Check sheet for the drawn part. Datum: minimum x, y, z corner. Units: mm. A direction names the side the tool comes from. Round coordinates to 2 decimals unless told otherwise and drop trailing zeros. Write each loop counter-clockwise with the first axis right and the second up, starting at its lowest first coordinate (ties: lowest second). Pieces come first, ordered by that corner, then holes. Notation, with made-up numbers: M 51.25,52.25 L 97.25,52.25 A23 cw 97.25,80.25 Z; hole C 49,58 d4. An arc over 180 degrees is marked long. One line per item, written item: value. Start each with the question number.
Item 1: Section check D-D, the plane x = 57.5. Record the cut outline in (y, z) (1 decimal).
Item 2: Section check C-C, the plane z = 24.5. Record the cut outline in (x, y), then the cut area to 3 significant figures.
Item 3: Thickness scan on probe 1 along Y at (x, z) = (97, 122); probe 2 along Z at (x, y) = (96, 33); probe 3 along X at (y, z) = (84, 38.5). Record the ranges inside material, lowest first. Write a range as from..to.
Item 4: Gauge pin test, flat ends, axial feed: pin 1 (10 mm diameter, centred on x = 66.5, y = 100.5, fed in from +Z); pin 2 (23 mm diameter, centred on x = 17.5, y = 20, fed in from -Z); pin 3 (5 mm diameter, centred on y = 39.5, z = 32.5, fed in from +X). Record the tip position at first contact, or that the pin passes through.
Item 5: Tool access check on the marked faces 1, 2, 3, 4 and 5. Record the directions out of +Z, -Z, +X, -X, +Y, -Y that give a thin tool (end or side, any length) a straight path to the whole face; none if there is none.
Item 6: Section check A-A, the plane x = 97.5. Record the cut outline in (y, z), then the cut area to 3 significant figures.
Item 7: Section check B-B, the plane y = 20. Record the cut outline in (x, z).
Item 8: Draft check along Y on the marked faces 6, 7 and 8. Enter one of: +Y half, -Y half, draft (parallel to the pull), parting line (faces both ways), or undercut.
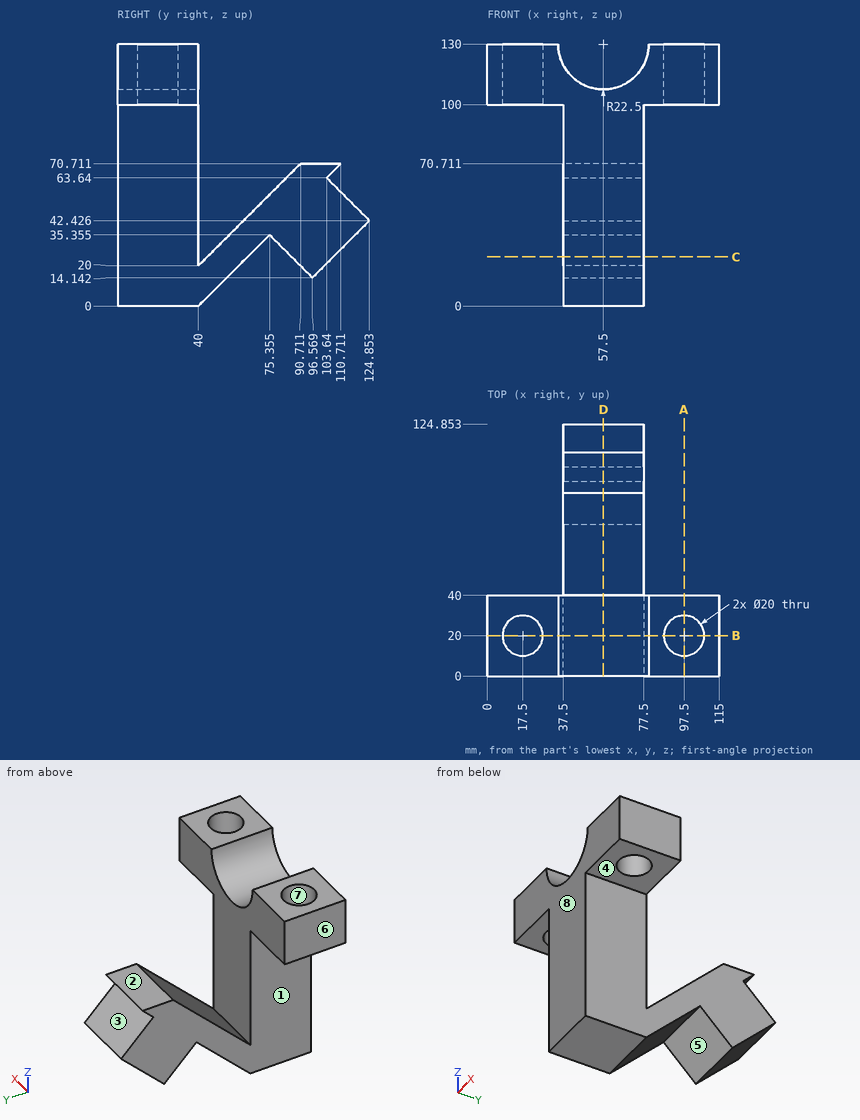
Response values:
1. outline: M 0,0 L 40,0 L 75.4,35.4 L 96.6,14.1 L 124.9,42.4 L 103.6,63.6 L 110.7,70.7 L 90.7,70.7 L 40,20 L 40,107.5 L 0,107.5 Z
2. outline: M 37.5,0 L 77.5,0 L 77.5,40 L 37.5,40 Z; M 37.5,44.5 L 77.5,44.5 L 77.5,64.5 L 37.5,64.5 Z; M 37.5,86.21 L 77.5,86.21 L 77.5,106.93 L 37.5,106.93 Z
2. area: 3,230 mm2
3. probe 1: y = 0..10.01, 29.99..40
3. probe 2: z = 100..130
3. probe 3: x = 37.5..77.5
4. pin 1: stops at z = 70.71
4. pin 2: stops at z = 100
4. pin 3: stops at x = 77.5
5. face 1: -Z, -X, +Y, -Y
5. face 2: +Z, +X, -X, +Y
5. face 3: +X, -X, +Y
5. face 4: -Z, +X, +Y, -Y
5. face 5: -Z, +X, -X
6. outline: M 0,100 L 10,100 L 10,130 L 0,130 Z; M 30,100 L 40,100 L 40,130 L 30,130 Z
6. area: 600 mm2
7. outline: M 0,100 L 7.5,100 L 7.5,130 L 0,130 Z; M 27.5,100 L 37.5,100 L 37.5,0 L 77.5,0 L 77.5,100 L 87.5,100 L 87.5,130 L 80,130 A22.5 cw 35,130 L 27.5,130 Z; M 107.5,100 L 115,100 L 115,130 L 107.5,130 Z
8. face 6: draft
8. face 7: undercut
8. face 8: -Y half
